```python
from build123d import *

# Parameters (mm, degrees)
SKETCH1_R           = 2.000000064
BOSS_EXTRUDE1_DEPTH = 152.4


with BuildPart() as part:
    # Sketch1 → Boss-Extrude1 (new, symmetric)
    with BuildSketch(Plane.XY):
        with BuildLine():
            ThreePointArc((4.181770846, 5.456960429), (3.437499983, 5.953924622), (2.634980936, 6.35))
            Line((2.634980936, 6.35), (-2.634980936, 6.35))
            ThreePointArc((-2.634980936, 6.35), (-3.437499983, 5.953924622), (-4.181770846, 5.456960429))
            Line((-4.181770846, 5.456960429), (-6.816751782, 0.893039571))
            ThreePointArc((-6.816751782, 0.893039571), (-6.874999966, 0), (-6.816751782, -0.893039571))
            Line((-6.816751782, -0.893039571), (-4.181770846, -5.456960429))
            ThreePointArc((-4.181770846, -5.456960429), (-3.437499983, -5.953924622), (-2.634980936, -6.35))
            Line((-2.634980936, -6.35), (2.634980936, -6.35))
            ThreePointArc((2.634980936, -6.35), (3.437499983, -5.953924622), (4.181770846, -5.456960429))
            Line((4.181770846, -5.456960429), (6.816751782, -0.893039571))
            ThreePointArc((6.816751782, -0.893039571), (6.860422465, -0.447468582), (6.874999966, 0))
            ThreePointArc((6.874999966, 0), (6.860422465, 0.447468582), (6.816751782, 0.893039571))
            Line((6.816751782, 0.893039571), (4.181770846, 5.456960429))
        make_face()
        with Locations(Location((0, 0, 0), (0, 0, 180))):
            Circle(SKETCH1_R, mode=Mode.SUBTRACT)
    extrude(amount=BOSS_EXTRUDE1_DEPTH, both=True)


solid = part.part
```
Geometry: final body of the model. Coordinates: model frame, mm. Coordinates: 2 decimals unless noted, no trailing zeros. Loops run counter-clockwise (first coordinate to the right, second up) from the corner with the lowest first, then second, coordinate; pieces in that order, holes last. Notation, with made-up numbers: (31.25, 79.25) -> (84.25, 79.25) arc R20 ccw to (84.25, 84.25) -> close; hole circle Ø6 at (11, 25). An arc over 180 degrees is marked (long way). Use a Markdown table: item, result. Add a question column.
(1) Pin query (flat end, axial travel): pin 1 Ø1 at (y, z) = (-3.5, -112) entering from -X. Return the tip coordinate at first contact, or that it passes through.
(2) Section query A-A, the plane z = 48. Return loops of the section in (x, y) (3 decimals), plus the area to 3 significant figures.
(3) Line query: line 1 along Y through (x, z) = (0, 73); line 2 along X through (y, z) = (0.25, -135); line 3 along X through (y, z) = (-1.5, 46). Output: solid intervals per line, ascending.
Answer:
| question | item | result |
|---|---|---|
| 1 | pin 1 | stops at x = -5.6 |
| 2 | outline | (-6.817, -0.893) -> (-4.182, -5.457) arc R6.875 ccw to (-2.635, -6.35) -> (2.635, -6.35) arc R6.875 ccw to (4.182, -5.457) -> (6.817, -0.893) arc R6.875 ccw to (6.817, 0.893) -> (4.182, 5.457) arc R6.875 ccw to (2.635, 6.35) -> (-2.635, 6.35) arc R6.875 ccw to (-4.182, 5.457) -> (-6.817, 0.893) arc R6.875 ccw to start; hole circle Ø4 at (0, 0) |
| 2 | area | 125 mm^2 |
| 3 | line 1 | y = -6.35 to -2, 2 to 6.35 |
| 3 | line 2 | x = -6.87 to -1.98, 1.98 to 6.87 |
| 3 | line 3 | x = -6.47 to -1.32, 1.32 to 6.47 |
